Could you check a few things on this drawing? It's one solid part, dimensions in mm from its lowest x, y, z. A direction names the side the tool comes from. Coordinates: 2 decimals unless noted, no trailing zeros. Loops run counter-clockwise (first coordinate to the right, second up) from the corner with the lowest first, then second, coordinate; pieces in that order, holes last. Notation, with made-up numbers: (54, 16) -> (81, 16) arc R17 cw to (81, 20) -> close; hole circle Ø2 at (-12, 79). An arc over 180 degrees is marked (long way). One line per question, with ' | ' between items.
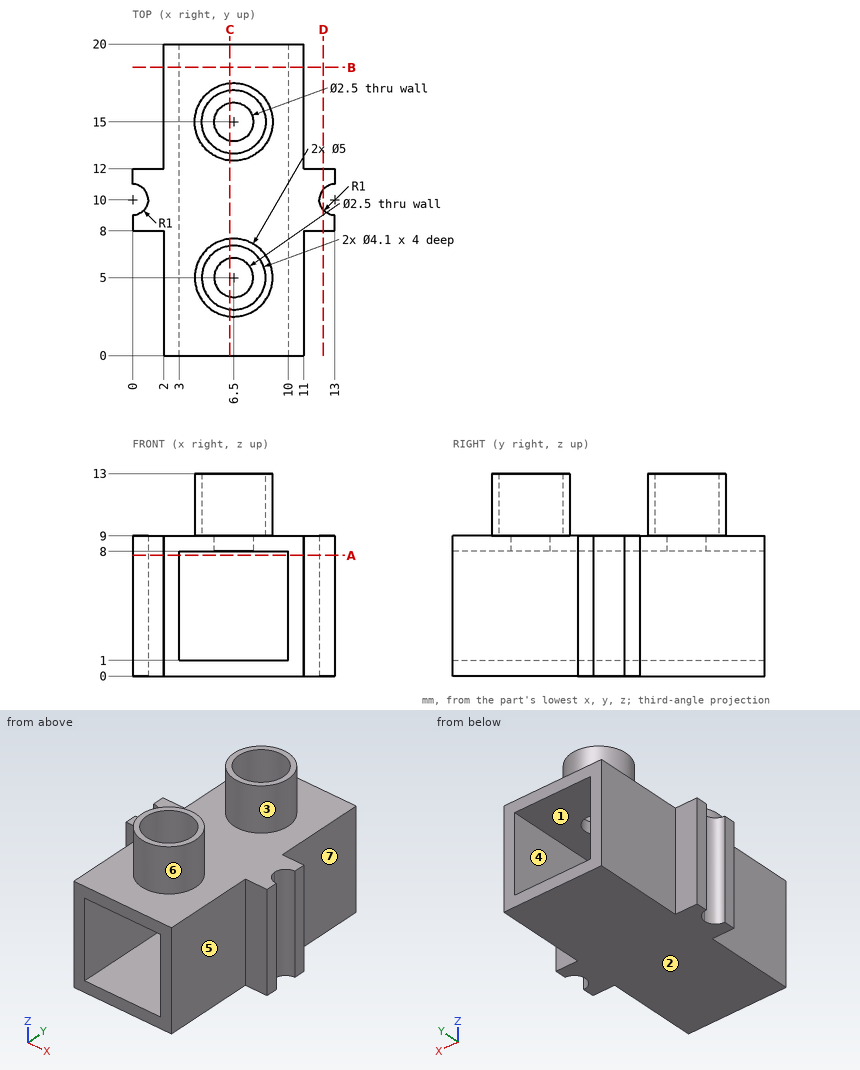
1) I need wall thicknesses on line 1 along Y through (x, z) = (6.5, 8.7); line 2 along Y through (x, z) = (6.5, 10.3); line 3 along Z through (x, y) = (3.5, 7.5). Which ranges of each line are inside material? Lowest first, please. Write a range as from..to.
Data:
line 1: 0..3.75, 6.25..13.75, 16.25..20 | line 2: 2.5..2.95, 7.05..7.5, 12.5..12.95, 17.05..17.5 | line 3: 0..1, 8..9
2) If we section it at A-A on z = 7.75: Please give me the cut outline in (x, y), and give its area (3 significant figures).
Data:
outline: (0, 8) -> (2, 8) -> (2, 0) -> (3, 0) -> (3, 20) -> (2, 20) -> (2, 12) -> (0, 12) -> (0, 11) arc R1 cw to (0, 9) -> close; (10, 0) -> (11, 0) -> (11, 8) -> (13, 8) -> (13, 9) arc R1 cw to (13, 11) -> (13, 12) -> (11, 12) -> (11, 20) -> (10, 20) -> close | area: 52.9 mm²
3) If we section it at D-D on x = 12.25: Please give me the cut outline in (y, z).
Data:
outline: (8, 0) -> (9.34, 0) -> (9.34, 9) -> (8, 9) -> close; (10.66, 0) -> (12, 0) -> (12, 9) -> (10.66, 9) -> close
4) We'd pull the mould along Z, two halves only. Please class the marked faces 1, 2 and 3: pulls with the +Z half, pulls with the -Z half, needs draft (parallel to the pull), parting line crosses it, or undercut.
Data:
face 1: undercut | face 2: pulls with the -Z half | face 3: needs draft
5) If we section it at C-C on x = 6.25: Give the number of separate pieces and of enclosed holes in the cut face, and give its area (3 significant figures).
Data:
separate pieces: 4 | enclosed holes: 0 | area: 42.3 mm²
6) If we section it at B-B on y = 18.5: Please give me the cut outline in (x, z), and give its area (3 significant figures).
Data:
outline: (2, 0) -> (11, 0) -> (11, 9) -> (2, 9) -> close; hole (3, 1) -> (10, 1) -> (10, 8) -> (3, 8) -> close | area: 32.0 mm²
7) I'm going to push flat-ended pins straight in: pin 1 Ø0.6 at (x, z) = (12, 5.5) entering from +Y; pin 2 Ø0.6 at (x, z) = (1.5, 2.5) entering from -Y; pin 3 Ø2 at (y, z) = (12, 10.5) entering from -X. Where does each tip first touch, or does it pass through?
Data:
pin 1: y = 12 | pin 2: y = 8 | pin 3: x = 5
8) On a 3-axis mill with a long thin cutter (end or side, diameter ignored), from which of +Z, -Z, +X, -X, +Y, -Y can I reach the whole of each face in a straight line? I mean the marked faces 4, 5, 6 and 7. Say none if no direction works.
Data:
face 4: +Y, -Y | face 5: +Z, -Z, +X, -Y | face 6: +Z | face 7: +Z, -Z, +X, +Y
